from build123d import *

# Parameters (mm, degrees)
SKETCH1_R           = 1.55
SKETCH1_R_2         = 4.5
BOSS_EXTRUDE1_DEPTH = 5
SKETCH2_R           = 3.5
CUT_EXTRUDE1_DEPTH  = 3


with BuildPart() as part:
    # Sketch1 → Boss-Extrude1 (new body)
    with BuildSketch(Plane.XY):
        with BuildLine():
            Line((-17.5, 4), (-11.842719282, 4))
            ThreePointArc((-11.842719282, 4), (0.007193328, 12.49999793), (11.847315168, 3.986367182))
            Line((11.847315168, 3.986367182), (17.170035324, 3.986367182))
            ThreePointArc((17.170035324, 3.986367182), (21.5, 0), (17.170035324, -3.986367182))
            Line((17.170035324, -3.986367182), (11.847315168, -3.986367182))
            ThreePointArc((11.847315168, -3.986367182), (0.007193328, -12.49999793), (-11.842719282, -4))
            Line((-11.842719282, -4), (-17.5, -4))
            ThreePointArc((-17.5, -4), (-21.5, 0), (-17.5, 4))
        make_face()
        with Locations((-17.5, 0)):
            Circle(SKETCH1_R, mode=Mode.SUBTRACT)
        with Locations((17.5, 0)):
            Circle(SKETCH1_R, mode=Mode.SUBTRACT)
        Circle(SKETCH1_R_2, mode=Mode.SUBTRACT)
        with Locations((0, 8.5)):
            Circle(SKETCH1_R, mode=Mode.SUBTRACT)
        with Locations((0, -8.5)):
            Circle(SKETCH1_R, mode=Mode.SUBTRACT)
    extrude(amount=BOSS_EXTRUDE1_DEPTH)

    # Sketch2 → Cut-Extrude1 (cut)
    with BuildSketch(Plane.XY.offset(5)):
        with Locations((0, 8.5)):
            Circle(SKETCH2_R)
        with Locations((0, -8.5)):
            Circle(SKETCH2_R)
    extrude(amount=-CUT_EXTRUDE1_DEPTH, mode=Mode.SUBTRACT)


solid = part.part
Part model, mm, in its own coordinate system. Give positions to 0.01 mm unless a question says otherwise; leave off trailing zeros. Order: outer loops, then holes, each group sorted by start corner. A loop starts at its lowest first (then second) coordinate and runs counter-clockwise, first axis right, second up. Notation, with made-up numbers: (-27, -18.75) - (-14, -18.75) arc R20 ccw to (-14, -2.75) - close; hole circle Ø2 at (-40, 15.5). An arc over 180 degrees is marked (long way). Use a Markdown table: item, result.
1) Saw through at B-B on y = 0. List the corners of the cut face in (x, z).
Checked values:
| item | result |
|---|---|
| outline | (-21.5, 0) - (-19.05, 0) - (-19.05, 5) - (-21.5, 5) - close; (-15.95, 0) - (-4.5, 0) - (-4.5, 5) - (-15.95, 5) - close; (4.5, 0) - (15.95, 0) - (15.95, 5) - (4.5, 5) - close; (19.05, 0) - (21.5, 0) - (21.5, 5) - (19.05, 5) - close |
2) Two-plate mould, pull along X, no slides. Class faces 1 (the cylindrical face through (-0.59, 4.46, 2.46)), 2 (the cylindrical face through (-19.05, 0.07, 2.46)), 3 (the cylindrical face through (-0.2, 12.5, 2.5)), 4 (the flat face through (-15, -4, 2)): +X half, -X half, draft (parallel to the pull), parting line (faces both ways), or undercut.
Checked values:
| item | result |
|---|---|
| face 1 | undercut |
| face 2 | undercut |
| face 3 | parting line |
| face 4 | draft |
3) Probe L1, parallel to Y at x = 0, z = 4; L2, parallel to Y at x = 0, z = 1.2; L3, parallel to X at y = 1, z = 2.55. List the from-to ranges inside material, lowest first. Write a range as from..to.
Checked values:
| item | result |
|---|---|
| L1 | -12.5..-12, -5..-4.5, 4.5..5, 12..12.5 |
| L2 | -12.5..-10.05, -6.95..-4.5, 4.5..6.95, 10.05..12.5 |
| L3 | -21.37..-18.68, -16.32..-4.39, 4.39..16.32, 18.68..21.37 |
4) Saw through at A-A on x = 0. List the corners of the cut face in (y, z).
Checked values:
| item | result |
|---|---|
| outline | (-12.5, 0) - (-10.05, 0) - (-10.05, 2) - (-12, 2) - (-12, 5) - (-12.5, 5) - close; (-6.95, 0) - (-4.5, 0) - (-4.5, 5) - (-5, 5) - (-5, 2) - (-6.95, 2) - close; (4.5, 0) - (6.95, 0) - (6.95, 2) - (5, 2) - (5, 5) - (4.5, 5) - close; (10.05, 0) - (12.5, 0) - (12.5, 5) - (12, 5) - (12, 2) - (10.05, 2) - close |
5) Saw through at D-D on y = 8.5. List the corners of the cut face in (x, z).
Checked values:
| item | result |
|---|---|
| outline | (-9.17, 0) - (-1.55, 0) - (-1.55, 2) - (-3.5, 2) - (-3.5, 5) - (-9.17, 5) - close; (1.55, 0) - (9.17, 0) - (9.17, 5) - (3.5, 5) - (3.5, 2) - (1.55, 2) - close |
6) Flat gauge pins, fed straight in: P1, Ø2, axis at x = 14.5, z = 2, coming from the +Y side; P2, Ø1, axis at y = 1, z = 1.5, coming from the +X side; P3, Ø3, axis at y = -9, z = 2, coming from the -X side; P4, Ø1.9, axis at x = -17.5, y = 0, coming from the +Z side. Where does each tip first touch, or does it go through?
Checked values:
| item | result |
|---|---|
| P1 | y = 3.99 |
| P2 | x = 21.47 |
| P3 | x = -10 |
| P4 | through |
7) Saw through at C-C on z = 4.3. List the corners of the cut face in (x, y).
Checked values:
| item | result |
|---|---|
| outline | (-17.5, -4) - (-11.84, -4) arc R12.5 ccw to (11.85, -3.99) - (17.17, -3.99) arc R4 ccw (long way) to (17.17, 3.99) - (11.85, 3.99) arc R12.5 ccw to (-11.84, 4) - (-17.5, 4) arc R4 ccw to start; hole circle Ø3.1 at (-17.5, 0); hole circle Ø9 at (0, 0); hole circle Ø7 at (0, -8.5); hole circle Ø7 at (0, 8.5); hole circle Ø3.1 at (17.5, 0) |
